Read the model definition and answer for the solid it produces. Units are mm, in the model's axes. A direction names the side the tool comes from. Round coordinates to 2 decimals unless told otherwise and drop trailing zeros. Order: outer loops, then holes, each group sorted by start corner. A loop starts at its lowest first (then second) coordinate and runs counter-clockwise, first axis right, second up.
from build123d import *

# Parameters (mm, degrees)
SKETCH1_R                = 2.75
BOSS_EXTRUDE1_DEPTH      = 5
BOSS_EXTRUDE1_DEPTH_BACK = 8
SKETCH2_R                = 3.952847075
BOSS_EXTRUDE2_DEPTH      = 4
SKETCH3_R                = 3.952847075
SKETCH3_R_2              = 2
BOSS_EXTRUDE3_DEPTH      = 2
FILLET1_R                = 1


with BuildPart() as part:
    # Sketch1 → Boss-Extrude1 (new body, two sides)
    with BuildSketch(Plane(origin=(0, 0, 255.707141652), x_dir=(-1, 0, 0), z_dir=(0, 0, -1))) as boss_extrude1_sk:
        with Locations((-95.862602529, 210.063080558)):
            Circle(SKETCH1_R)
    extrude(amount=BOSS_EXTRUDE1_DEPTH)
    extrude(boss_extrude1_sk.sketch, amount=-BOSS_EXTRUDE1_DEPTH_BACK)

    # Sketch2 → Boss-Extrude2 (add)
    with BuildSketch(Plane(origin=(0, 0, 250.707141652), x_dir=(-1, 0, 0), z_dir=(0, 0, -1))):
        with Locations((-95.862602529, 210.063080558)):
            Circle(SKETCH2_R)
    extrude(amount=BOSS_EXTRUDE2_DEPTH)

    # Sketch3 → Boss-Extrude3 (add)
    with BuildSketch(Plane(origin=(0, 0, 246.707141652), x_dir=(-1, 0, 0), z_dir=(0, 0, -1))):
        with Locations((-95.862602529, 210.063080558)):
            Circle(SKETCH3_R)
        with Locations((-95.862602529, 210.063080558)):
            Circle(SKETCH3_R_2, mode=Mode.SUBTRACT)
    extrude(amount=BOSS_EXTRUDE3_DEPTH)

    # Fillet1
    fillet1_edges = [part.edges().sort_by_distance(p)[0] for p in [
        (98.612602529, 210.063080558, 263.707141652),
    ]]
    fillet(fillet1_edges, radius=FILLET1_R)


solid = part.part
Q1. A cutting plane is placed at C-C, the plane z = 258.5. Give the vertices of the cut face in (x, y), plus the area to 3 significant figures.
Outcome:
outline: circle Ø5.5 at (95.86, 210.06)
area: 23.8 mm2
Q2. A cutting plane is placed at B-B, the plane x = 92.5. Give the vertices of the cut face in (y, z).
Outcome:
outline: (207.99, 244.71) - (212.14, 244.71) - (212.14, 250.71) - (207.99, 250.71) - close
Q3. For a pull along X with two mould halves and no side action, classify faces 3 (the face through (94.38, 212.38, 256.62)), 4 (the face through (95, 213, 250.707)), 5 (the face through (96.123, 212.046, 245.721)) as released by +X, released by -X, zero draft, split by the parting line, or undercut.
Outcome:
face 3: split by the parting line
face 4: zero draft
face 5: undercut
Q4. Straight lines are drawn through the part: probe 1 along Z at (x, y) = (94.5, 213); probe 2 along Y at (x, z) = (95.75, 253.75); probe 3 along X at (y, z) = (211.75, 257.5). For each, find the intervals that lie inside material, in ascending order.
Outcome:
probe 1: z = 244.71 to 250.71
probe 2: y = 207.32 to 212.81
probe 3: x = 93.69 to 98.03
Q5. For faces 1 (the face through (96, 210, 246.707)), 2 (the face through (97, 212, 244.707)), determine the directions among +Z, -Z, +X, -X, +Y, -Y from which every point of the face is accessible in a straight line to the end or side of a thin tool.
Outcome:
face 1: -Z
face 2: -Z, +X, -X, +Y, -Y
Q6. A cutting plane is placed at D-D, the plane z = 249.25. Give the vertices of the cut face in (x, y), plus the area to 3 significant figures.
Outcome:
outline: circle Ø7.91 at (95.86, 210.06)
area: 49.1 mm2
Q7. A cutting plane is placed at A-A, the plane z = 246.5. Give the vertices of the cut face in (x, y).
Outcome:
outline: circle Ø7.91 at (95.86, 210.06); hole circle Ø4 at (95.86, 210.06)
Q8. Flat-ended cylindrical pins translate along their axes: pin 1 (4 mm diameter, centred on x = 93, y = 207.5, fed in from +Z); pin 2 (1.5 mm diameter, centred on y = 209, z = 259.5, fed in from -X); pin 3 (1.2 mm diameter, centred on x = 95.5, y = 210.5, fed in from -Z). Find the tip coordinate at first contact, or state that the pin passes through.
Outcome:
pin 1: stops at z = 263.7
pin 2: stops at x = 93.13
pin 3: stops at z = 246.71
